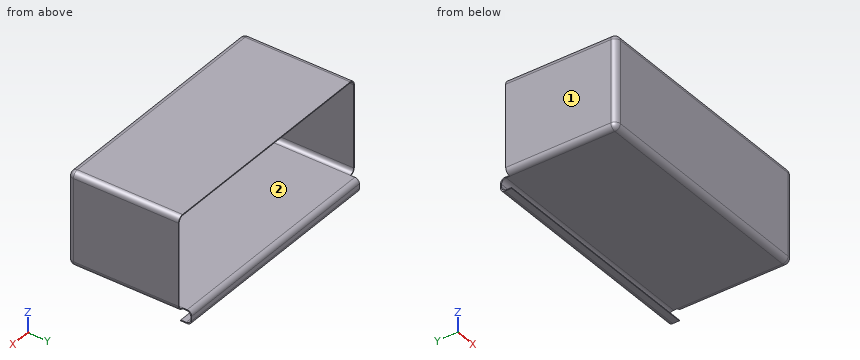
from build123d import *

# Parameters (mm, degrees)
SKETCH1_W           = 260
SKETCH1_H           = 100
BOSS_EXTRUDE1_DEPTH = 120
FILLET1_R           = 5
SHELL1_T            = 1


with BuildPart() as part:
    # Sketch1 → Boss-Extrude1 (new body)
    with BuildSketch(Plane(origin=(0, 0, 0), x_dir=(1, 0, 0), z_dir=(0, 1, 0))):
        Rectangle(SKETCH1_W, SKETCH1_H)
    extrude(amount=-BOSS_EXTRUDE1_DEPTH)

    # Fillet1
    fillet1_edges = [part.edges().sort_by_distance(p)[0] for p in [
        (130, -120, 0),
        (0, -120, -50),
        (-130, -120, 0),
        (-130, -60, -50),
        (130, -60, -50),
        (130, -60, 50),
        (-130, -60, 50),
        (0, -120, 50),
    ]]
    fillet(fillet1_edges, radius=FILLET1_R)

    # Shell1
    shell1_openings = [part.faces().sort_by_distance(p)[0] for p in [
        (0, 0, 0),
    ]]
    offset(amount=SHELL1_T, openings=shell1_openings, kind=Kind.INTERSECTION)

    # Sweep1: sweep along a path in Sketch3
    with BuildLine(Plane(origin=(0, 0, 0), x_dir=(1, 0, 0), z_dir=(0, 1, 0))) as sweep1_path:
        Line((-125, 51), (125, 51))
    # Sketch2 → Sweep1 (sweep)
    with BuildSketch(Plane(origin=(0, 0, 0), x_dir=(0, 0, -1), z_dir=(1, 0, 0))):
        with BuildLine():
            Line((51, 0), (51, 4))
            ThreePointArc((51, 4), (52.464466094, 7.535533906), (56, 9))
            Line((56, 9), (59, 9))
            ThreePointArc((59, 9), (62.535533906, 7.535533906), (64, 4))
            Line((64, 4), (64, -2))
            Line((64, -2), (65, -2))
            Line((65, -2), (65, 5))
            ThreePointArc((65, 5), (63.535533906, 8.535533906), (60, 10))
            Line((60, 10), (55, 10))
            ThreePointArc((55, 10), (51.464466094, 8.535533906), (50, 5))
            Line((50, 5), (50, 0))
            Line((50, 0), (51, 0))
        make_face()
    sweep(path=sweep1_path.line)


solid = part.part
Check sheet for the modelled part. Datum: model origin and axes. Units: mm. Face numbers are marked on the shaded views. A direction names the side the tool comes from. Give positions to 0.01 mm unless a question says otherwise; leave off trailing zeros. Loops run counter-clockwise (first coordinate to the right, second up) from the corner with the lowest first, then second, coordinate; pieces in that order, holes last. Notation, with made-up numbers: M 6.25,-22 L 13.25,-22 A18 ccw 13.25,-14 Z; hole C -20.75,-12 d5. An arc over 180 degrees is marked long. Answer as a JSON object with one key per item and string values. Group by question number.
Q1. Access from +Z, -Z, +X, -X, +Y, -Y to the whole of each face (thin tool, end or side, straight path). Record for the marked faces 1 and 2.
Q2. Cross-section at A-A on y = -68. Record the cut outline in (x, z), then the cut area to 3 significant figures.
Q3. Go/stop test with flat-tipped pins: P1, Ø4, axis at x = -38.5, z = -46.5, coming from the +Y side; P2, Ø13, axis at y = 7, z = -60.5, coming from the +X side; P3, Ø3.5, axis at y = 6.5, z = -60, coming from the -X side; P4, Ø8, axis at x = -81.5, y = -78, coming from the -Z side. Record where each tip stops, or that it passes through.
Q4. Cross-section at C-C on z = 13.5. Record the cut outline in (x, y).
Q5. Material ranges on line 1 along X through (y, z) = (-77, -29); line 2 along Z through (x, y) = (-102.5, -40); line 3 along Z through (x, y) = (-3, 2.5), recorded low to high. Write a range as [from, to].
Q6. Cross-section at B-B on x = 43. Record the cut outline in (y, z), then the cut area to 3 significant figures.
Evaluation:
{
 "1": {"face 1": "+Z, -Z, -X, +Y, -Y", "face 2": "+Y"},
 "2": {"outline": "M -131,-45 A6 ccw -125,-51 L 125,-51 A6 ccw 131,-45 L 131,45 A6 ccw 125,51 L -125,51 A6 ccw -131,45 Z; hole M -130,-45 A5 ccw -125,-50 L 125,-50 A5 ccw 130,-45 L 130,45 A5 ccw 125,50 L -125,50 A5 ccw -130,45 Z", "area": "715 mm2"},
 "3": {"P1": "stops at y = -118.57", "P2": "stops at x = 125", "P3": "passes through", "P4": "stops at z = -51"},
 "4": {"outline": "M -131,-115 A6 ccw -125,-121 L 125,-121 A6 ccw 131,-115 L 131,0 L 130,0 L 130,-115 A5 cw 125,-120 L -125,-120 A5 cw -130,-115 L -130,0 L -131,0 Z"},
 "5": {"line 1": "x = [-131, -130], [130, 131]", "line 2": "z = [-51, -50], [50, 51]", "line 3": "z = [-65, -64], [-51, -50]"},
 "6": {"outline": "M -121,-45 A6 ccw -115,-51 L 4,-51 A5 cw 9,-56 L 9,-59 A5 cw 4,-64 L -2,-64 L -2,-65 L 5,-65 A5 ccw 10,-60 L 10,-55 A5 ccw 5,-50 L -115,-50 A5 cw -120,-45 L -120,45 A5 cw -115,50 L 0,50 L 0,51 L -115,51 A6 ccw -121,45 Z", "area": "372 mm2"}
}
